Design review of the part built by this model. Coordinates are the model's own, in mm. Give positions to 0.01 mm unless a question says otherwise; leave off trailing zeros. Order: outer loops, then holes, each group sorted by start corner. A loop starts at its lowest first (then second) coordinate and runs counter-clockwise, first axis right, second up. Notation, with made-up numbers: (24.5, 61) -> (52.5, 61) arc R31 cw to (52.5, 97) -> close; hole circle Ø10 at (43.25, 6). An arc over 180 degrees is marked (long way). Use a Markdown table: item, result. Add a question column.
Autodesk Inventor part; units mm, degrees
ref_plane "YZ Plane" through (0, 0, 0) normal (1, 0, 0) x (0, 1, 0)
ref_plane "XZ Plane" through (0, 0, 0) normal (0, 1, 0) x (-1, 0, 0)
ref_plane "XY Plane" through (0, 0, 0) normal (0, 0, 1) x (1, 0, 0)
sketch "Эскиз1" plane through (0, 0, 0) normal (0, 0, 1) x (1, 0, 0)
  circle A0 centre (0, 0) radius 30.75
  circle A1 centre (24, -24) radius 1.5
  circle A2 centre (24, 24) radius 1.5
  circle A3 centre (-24, 24) radius 1.5
  circle A4 centre (-24, -24) radius 1.5
  line L0 (-78, 42.5) -> (-75, 42.5)
  line L1 (-75, 32.5) -> (-78, 32.5)
  line L2 (-78, 32.5) -> (-78, 42.5)
  line L3 (-78, 5) -> (-75, 5)
  line L4 (-78, 0) -> (-78, 5)
  line L5 (-42.5, 78) -> (-32.5, 78)
  line L6 (-32.5, 78) -> (-32.5, 75)
  line L7 (-42.5, 75) -> (-42.5, 78)
  line L8 (-5, 78) -> (0, 78)
  line L9 (-5, 75) -> (-5, 78)
  line L10 (-5, 75) -> (-32.5, 75)
  line L11 (-42.5, 75) -> (-75, 75)
  line L12 (-75, 75) -> (-75, 42.5)
  line L13 (-75, 32.5) -> (-75, 5)
  line L14 (78, 42.5) -> (75, 42.5)
  line L15 (75, 32.5) -> (78, 32.5)
  line L16 (78, 32.5) -> (78, 42.5)
  line L17 (78, 5) -> (75, 5)
  line L18 (78, 0) -> (78, 5)
  line L19 (42.5, 78) -> (32.5, 78)
  line L20 (32.5, 78) -> (32.5, 75)
  line L21 (42.5, 75) -> (42.5, 78)
  line L22 (5, 78) -> (0, 78)
  line L23 (5, 75) -> (5, 78)
  line L24 (5, 75) -> (32.5, 75)
  line L25 (42.5, 75) -> (75, 75)
  line L26 (75, 5) -> (75, 32.5)
  line L27 (75, 75) -> (75, 42.5)
  line L28 (-78, -42.5) -> (-75, -42.5)
  line L29 (-75, -32.5) -> (-78, -32.5)
  line L30 (-78, -32.5) -> (-78, -42.5)
  line L31 (-78, -5) -> (-75, -5)
  line L32 (-78, 0) -> (-78, -5)
  line L33 (-42.5, -78) -> (-32.5, -78)
  line L34 (-32.5, -78) -> (-32.5, -75)
  line L35 (-42.5, -75) -> (-42.5, -78)
  line L36 (-5, -78) -> (0, -78)
  line L37 (-5, -75) -> (-5, -78)
  line L38 (-5, -75) -> (-32.5, -75)
  line L39 (-42.5, -75) -> (-75, -75)
  line L40 (-75, -5) -> (-75, -32.5)
  line L41 (-75, -75) -> (-75, -42.5)
  line L42 (75, -32.5) -> (78, -32.5)
  line L43 (75, -32.5) -> (75, -5)
  line L44 (78, -5) -> (75, -5)
  line L45 (78, 0) -> (78, -5)
  line L46 (78, -42.5) -> (75, -42.5)
  line L47 (78, -32.5) -> (78, -42.5)
  line L48 (5, -75) -> (32.5, -75)
  line L49 (5, -78) -> (0, -78)
  line L50 (5, -75) -> (5, -78)
  line L51 (75, -42.5) -> (75, -75)
  line L52 (42.5, -75) -> (75, -75)
  line L53 (32.5, -78) -> (32.5, -75)
  line L54 (42.5, -78) -> (32.5, -78)
  line L55 (42.5, -75) -> (42.5, -78)
extrude "Выдавливание1" add sketch "Эскиз1" along normal blind 3
properties part number "Верх"
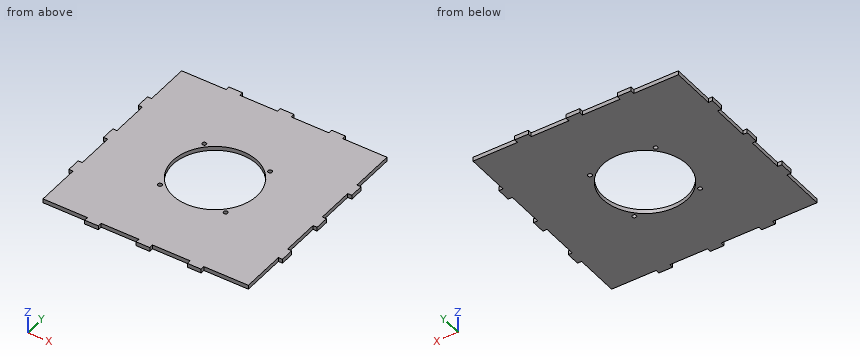
1) Add section A-A (x = 0). Give the boundary of the cut face in (y, z), then the cut area to 4 significant figures.
2) For L1, parallel to Y at x = 24, z = 2.05; L2, parallel to Y at x = 50, z = 0.5; L3, parallel to Y at x = -2, z = 0.6, list the stretches that pass through material, from the lowest coordinate up. Write a range as [from, to].
3) Add section C-C (z = 0.55). Give the number of separate pieces and of enclosed holes in the cut face, then the cut area to 3 significant figures.
4) Add section D-D (x = 44.5). Give the boundary of the cut face in (y, z).
5) Insertion check: pin 1 (0.9 mm diameter, centred on y = -76.5, z = 2, fed in from +X); pin 2 (0.9 mm diameter, centred on y = -77, z = 1.5, fed in from -X); pin 3 (1.5 mm diameter, centred on x = -21.5, z = 2, fed in from -Y). Each pin has a flat end and moves straight along its axis. Give the tip position at first contact, or say it passes through.
Worked answers:
| question | item | result |
|---|---|---|
| 1 | outline | (-78, 0) -> (-30.75, 0) -> (-30.75, 3) -> (-78, 3) -> close; (30.75, 0) -> (78, 0) -> (78, 3) -> (30.75, 3) -> close |
| 1 | area | 283.5 mm^2 |
| 2 | L1 | [-75, -25.5], [-22.5, -19.22], [19.22, 22.5], [25.5, 75] |
| 2 | L2 | [-75, 75] |
| 2 | L3 | [-78, -30.68], [30.68, 78] |
| 3 | separate pieces | 1 |
| 3 | enclosed holes | 5 |
| 3 | area | 19,900 mm^2 |
| 4 | outline | (-75, 0) -> (75, 0) -> (75, 3) -> (-75, 3) -> close |
| 5 | pin 1 | x = 42.5 |
| 5 | pin 2 | x = -42.5 |
| 5 | pin 3 | y = -75 |
